For this review, take the finished solid that the model builds, in its own axes (mm). A direction names the side the tool comes from. Round coordinates to 2 decimals unless told otherwise and drop trailing zeros. Order: outer loops, then holes, each group sorted by start corner. A loop starts at its lowest first (then second) coordinate and runs counter-clockwise, first axis right, second up.
from build123d import *

# Parameters (mm, degrees)
F1_DEPTH = 2
F2_DEPTH = 25
F3_R     = 1.5
F4_DEPTH = 34
F5_DEPTH = 34


with BuildPart() as f1:
    # F0 (on Top) → F1 (new body)
    with BuildSketch(Plane.XY):
        Polygon((0, -15), (20, -15), (20, 15), (0, 15), (-20, 15), (-20, -15), align=None)
    extrude(amount=F1_DEPTH)

    # F0 (on Top) → F2 (join)
    with BuildSketch(Plane.XY):
        Polygon((0, 15), (20, 15), (20, 17), (-20, 17), (-20, 15), align=None)
        Polygon((-20, -17), (20, -17), (20, -15), (0, -15), (-20, -15), align=None)
    extrude(amount=F2_DEPTH)

    # F3 (on face) → F4 (cut)
    with BuildSketch(Plane.XZ.offset(17)):
        with BuildLine():
            ThreePointArc((-20, 17), (-17.656854, 22.656854), (-12, 25))
            Line((-12, 25), (-20, 25))
            Line((-20, 25), (-20, 17))
        make_face()
        with Locations((-10, 21)):
            Circle(F3_R)
    extrude(amount=-F4_DEPTH, mode=Mode.SUBTRACT)

    # F3 (on face) → F5 (join)
    with BuildSketch(Plane.XZ.offset(17)):
        Polygon((20, 25), (17.921008, 25), (12.244668, 5), (14.32366, 5), align=None)
        Polygon((23.133647, 43.366198), (17.921008, 25), (20, 25), (25.212639, 43.366198), align=None)
    extrude(amount=-F5_DEPTH)


solid = f1.part
(1) Clearance check with flat-ended pins moving along their axes: P1, Ø4, axis at y = 12.5, z = 33.5, coming from the -X side; P2, Ø9, axis at x = 1.5, y = 0, coming from the +Z side; P3, Ø1.6, axis at x = 4, y = -15.5, coming from the +Z side; P4, Ø2.5, axis at x = -10, z = 21, coming from the -Y side. State where each tip first meets the part, or that it passes through.
(2) Add section D-D on x = 0. Give the boundary of the cut face in (y, z), plus the area to 3 significant figures.
(3) Add section A-A on y = 12. Give the boundary of the cut face in (x, z), plus the area to 3 significant figures.
(4) Add section C-C on z = 21. Give the boundary of the cut face in (x, y).
(5) Wall thickness on L1, parallel to Z at x = -10, y = -16.5; L2, parallel to Y at x = 5, z = 24; L3, parallel to Z at x = -17, y = 1: over which ranges is each line inside the solid? List them lowest first.
(6) Draft analysis for pull direction Z (two halves, no side actions). For faces 4 (the face through (-11.11, -16.01, 22.01)), 5 (the face through (-17.719, 15.986, 22.594)), 6 (the face through (2, -17, 12)), state which applies: pulls with the +Z half, pulls with the -Z half, needs draft (parallel to the pull), parting line crosses it, or undercut.
(7) Add section B-B on x = -10. Give the boundary of the cut face in (y, z).
(8) Tool access review of faces 1 (the face through (13, 0, 5)), 2 (the face through (3, -16, 25)), 3 (the face through (20, -3, 1)): name each direction out of +Z, -Z, +X, -X, +Y, -Y from which nothing blocks a thin tool from reaching the whole face with its end or side.
Here are the results:
1. P1: stops at x = 19.77
1. P2: stops at z = 2
1. P3: stops at z = 25
1. P4: passes through
2. outline: (-17, 0) - (17, 0) - (17, 25) - (15, 25) - (15, 2) - (-15, 2) - (-15, 25) - (-17, 25) - close
2. area: 160 mm2
3. outline: (-20, 0) - (20, 0) - (20, 2) - (-20, 2) - close; (12.24, 5) - (14.32, 5) - (25.21, 43.37) - (23.13, 43.37) - close
3. area: 160 mm2
4. outline: (-18.93, -17) - (-11.5, -17) - (-11.5, -15) - (-18.93, -15) - close; (-18.93, 15) - (-11.5, 15) - (-11.5, 17) - (-18.93, 17) - close; (-8.5, -17) - (20, -17) - (20, -15) - (18.86, -15) - (18.86, 15) - (20, 15) - (20, 17) - (-8.5, 17) - (-8.5, 15) - (16.79, 15) - (16.79, -15) - (-8.5, -15) - close
5. L1: z = 0 to 19.5, 22.5 to 25
5. L2: y = -17 to -15, 15 to 17
5. L3: z = 0 to 2
6. face 4: undercut
6. face 5: pulls with the +Z half
6. face 6: needs draft
7. outline: (-17, 0) - (17, 0) - (17, 19.5) - (15, 19.5) - (15, 2) - (-15, 2) - (-15, 19.5) - (-17, 19.5) - close; (-17, 22.5) - (-15, 22.5) - (-15, 25) - (-17, 25) - close; (15, 22.5) - (17, 22.5) - (17, 25) - (15, 25) - close
8. face 1: +X, -X
8. face 2: +Z, -X, +Y, -Y
8. face 3: -Z, +X, +Y, -Y
